Here's the drawing with two shaded views (mm, measured from the low corner). I have some questions. A direction names the side the tool comes from. Give positions to 0.01 mm unless a question says otherwise; leave off trailing zeros. Loops run counter-clockwise (first coordinate to the right, second up) from the corner with the lowest first, then second, coordinate; pieces in that order, holes last. Notation, with made-up numbers: (77.25, -30) - (96.25, -30) arc R10 cw to (96.25, -26) - close; hole circle Ø6 at (31, 20). An arc over 180 degrees is marked (long way). Answer as a JSON object with one key per item and string values. Group by question number.
Item 1: Please list where these lines run through material, in increasing order: L1, parallel to Y at x = 38, z = 7; L2, parallel to X at y = 101.6, z = 4; L3, parallel to X at y = 118, z = 26.5.
Item 2: Will this pin go through, and if not, where does the flat tip stop? pin 1 (6 mm diameter, centred on x = 14.5, y = 39, fed in from +Z).
Item 3: Suppose I cut it at B-B on x = 38.1. Write out the boundary of the cut face in (y, z), and give its area (3 significant figures).
Item 4: Suppose I cut it at D-D on x = 81. Write out the boundary of the cut face in (y, z).
Item 5: Which directions (+Z, -Z, +X, -X, +Y, -Y) give clear straight access to the entire face, cutting with the end or side of a thin tool? Please do the marked faces 4 and 5.
Item 6: Suppose I cut it at A-A on y = 101.6. Write out the boundary of the cut face in (x, z).
Item 7: Thinking about a two-plate mould opening in X: for the marked faces 1, 2 and 3, which applies, pulls with the +X half, pulls with the -X half, needs draft (parallel to the pull), parting line crosses it, or undercut?
Item 8: Suppose I cut it at C-C on z = 65.5. Write out the boundary of the cut face in (x, y), and give its area (3 significant figures).
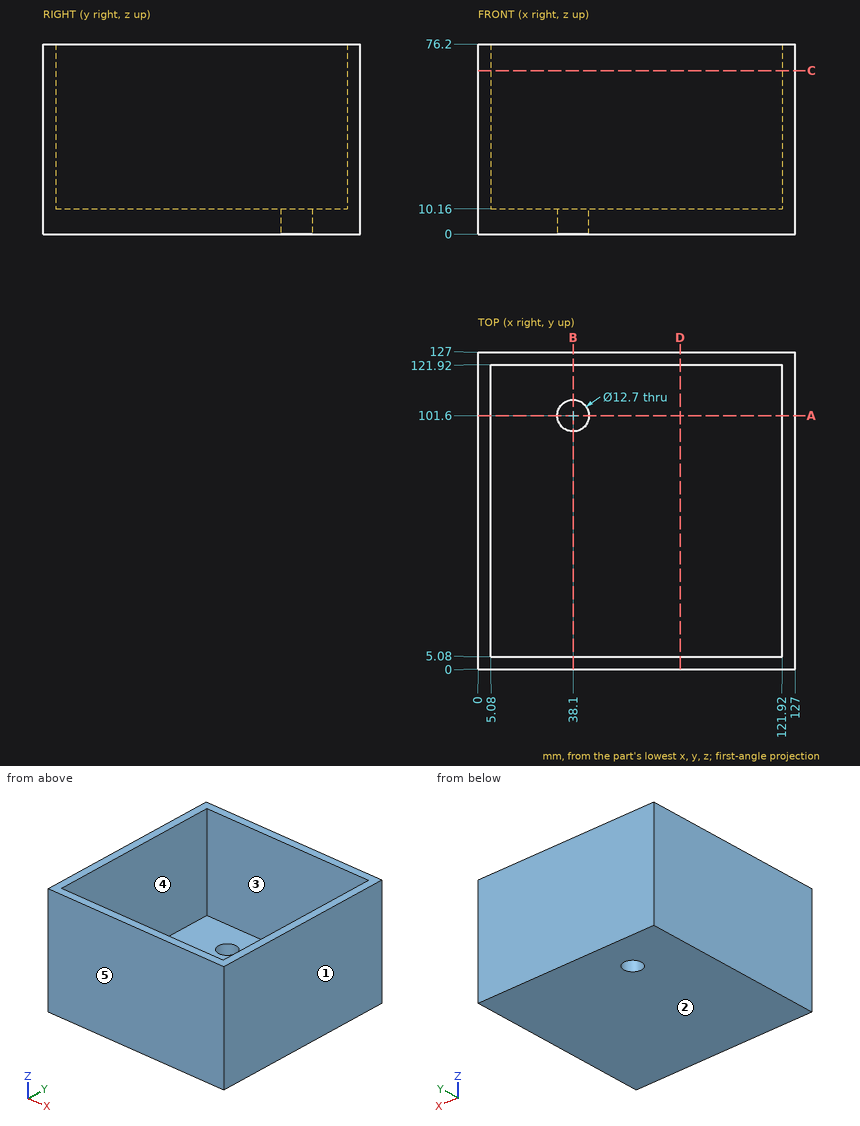
Worked out:
{
 "1": {"L1": "y = 0 to 95.25, 107.95 to 127", "L2": "x = 0 to 31.75, 44.45 to 127", "L3": "x = 0 to 5.08, 121.92 to 127"},
 "2": {"pin 1": "stops at z = 10.16"},
 "3": {"outline": "(0, 0) - (95.25, 0) - (95.25, 10.16) - (5.08, 10.16) - (5.08, 76.2) - (0, 76.2) - close; (107.95, 0) - (127, 0) - (127, 76.2) - (121.92, 76.2) - (121.92, 10.16) - (107.95, 10.16) - close", "area": "1,830 mm2"},
 "4": {"outline": "(0, 0) - (127, 0) - (127, 76.2) - (121.92, 76.2) - (121.92, 10.16) - (5.08, 10.16) - (5.08, 76.2) - (0, 76.2) - close"},
 "5": {"face 4": "+Z", "face 5": "+Z, -Z, +X, -X, -Y"},
 "6": {"outline": "(0, 0) - (31.75, 0) - (31.75, 10.16) - (5.08, 10.16) - (5.08, 76.2) - (0, 76.2) - close; (44.45, 0) - (127, 0) - (127, 76.2) - (121.92, 76.2) - (121.92, 10.16) - (44.45, 10.16) - close"},
 "7": {"face 1": "pulls with the +X half", "face 2": "needs draft", "face 3": "undercut"},
 "8": {"outline": "(0, 0) - (127, 0) - (127, 127) - (0, 127) - close; hole (5.08, 5.08) - (121.92, 5.08) - (121.92, 121.92) - (5.08, 121.92) - close", "area": "2,480 mm2"}
}
